Part print with two shaded views. Sizes in mm from the minimum x, y, z corner. A direction names the side the tool comes from. Give positions to 0.01 mm unless a question says otherwise; leave off trailing zeros. Write each loop counter-clockwise with the first axis right and the second up, starting at its lowest first coordinate (ties: lowest second). Pieces come first, ordered by that corner, then holes. Notation, with made-up numbers: (-19, 43) - (-8, 43) arc R23 cw to (-8, 68) - close; hole circle Ø2 at (-35, 13.25). An arc over 180 degrees is marked (long way). One line per item, written item: value. Start each with the question number.
(1) 3-axis set-ups, long thin cutter, end or side, ignore diameter. For the marked faces 4, 5, 6 and 7: which of +Z, -Z, +X, -X, +Y, -Y reach the whole face in a straight line?
(2) Probe L1, parallel to X at y = 15.75, z = 0.75; L2, parallel to X at y = 14.5, z = 2.75; L3, parallel to Y at x = 2.5, z = 3.5. List the from-to ranges inside material, lowest first.
(3) Drop flat-ended pins along their axis: P1, Ø0.6, axis at x = 4, y = 2.5, coming from the -Z side; P2, Ø1, axis at x = 3.5, y = 7, coming from the -Z side; P3, Ø3.5, axis at x = 7, y = 11, coming from the +Z side; P4, Ø3, axis at y = 6.5, z = 7, coming from the +X side. Give the stop position or say it passes through.
(4) Mould opens along X. For the marked faces 1, 2 and 3 say: pulls with the +X half, pulls with the -X half, needs draft (parallel to the pull), parting line crosses it, or undercut.
(5) Cut at C-C, the plane y = 9. List the corners of the cut face in (x, z).
(6) Cut at A-A, the plane z = 1.5. List the corners of the cut face in (x, y).
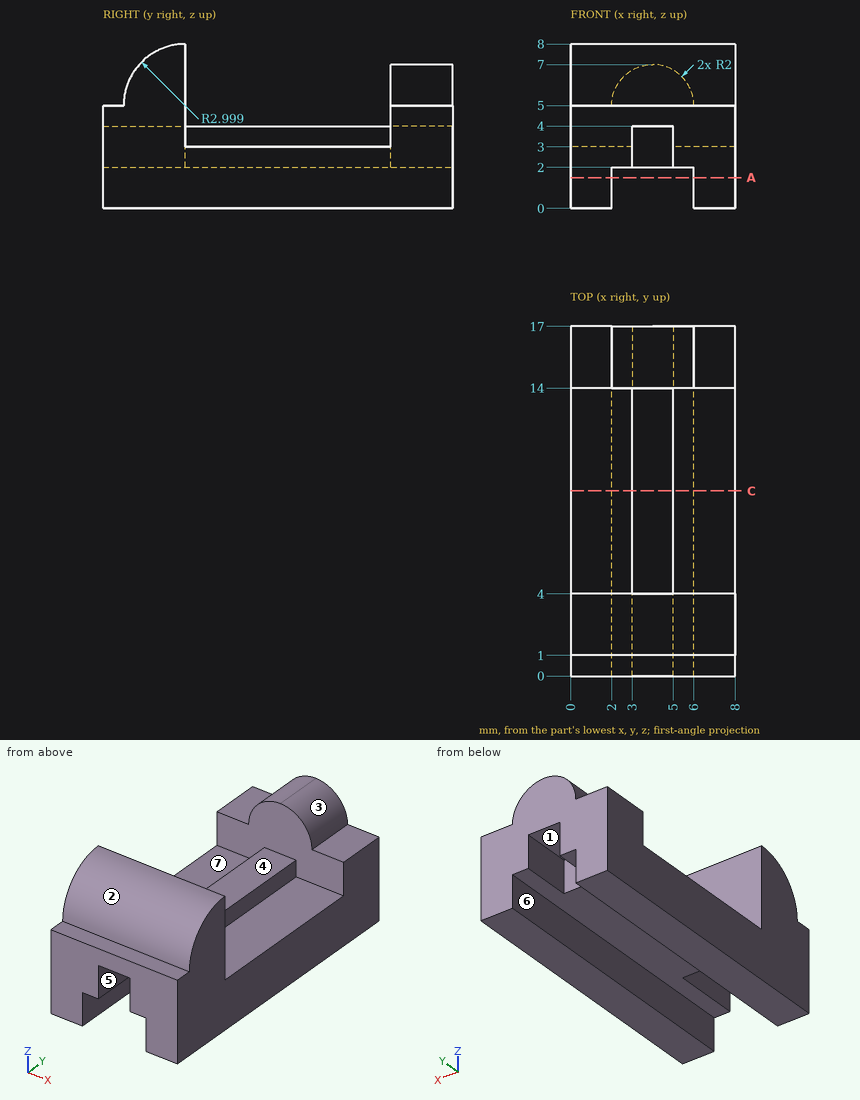
Answers follow:
1. face 4: +Z, +X, -X
1. face 5: -Z, -Y
1. face 6: -Z, +Y, -Y
1. face 7: +Z, -X
2. L1: x = 0 to 2, 6 to 8
2. L2: x = 0 to 3, 5 to 8
2. L3: y = 0 to 4, 14 to 17
3. P1: stops at z = 4
3. P2: stops at z = 2
3. P3: stops at z = 3
3. P4: passes through
4. face 1: undercut
4. face 2: needs draft
4. face 3: pulls with the +X half
5. outline: (0, 0) - (2, 0) - (2, 2) - (6, 2) - (6, 0) - (8, 0) - (8, 3) - (5, 3) - (5, 4) - (3, 4) - (3, 3) - (0, 3) - close
6. outline: (0, 0) - (2, 0) - (2, 17) - (0, 17) - close; (6, 0) - (8, 0) - (8, 17) - (6, 17) - close
